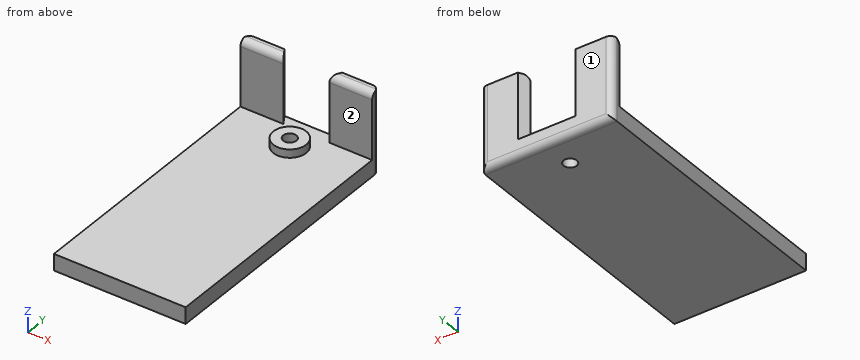
Autodesk Inventor part; units mm, degrees
ref_plane "YZ Plane" through (0, 0, 0) normal (1, 0, 0) x (0, 1, 0)
ref_plane "XZ Plane" through (0, 0, 0) normal (0, 1, 0) x (-1, 0, 0)
ref_plane "XY Plane" through (0, 0, 0) normal (0, 0, 1) x (1, 0, 0)
sketch "Skizze1" plane through (0, 0, 0) normal (0, 0, 1) x (1, 0, 0)
  line L0 (-20, 15) -> (20, 15)
  line L1 (20, 15) -> (20, -67)
  line L2 (20, -67) -> (-20, -67)
  line L3 (-20, -67) -> (-20, 15)
  line L4 (0, -83.4) -> (0, 31.4)
  point P0 (0, 0)
  point P1 (0, 15)
  dimension "d2" = 82
  dimension "d4" = 15
  dimension "d42" = 40
extrude "Extrusion1" add sketch "Skizze1" along normal blind 5
sketch "Skizze2" plane through (0, 0, 5) normal (0, 0, 1) x (1, 0, 0)
  line L0 (20, 15) -> (-20, 15)
  circle A0 centre (0, 5) radius 5
  line L1 (0, -83.4) -> (0, 31.4)
  point P0 (0, 0)
  dimension "d10" = 10
  dimension "d11" = 10
extrude "Extrusion2" add sketch "Skizze2" along normal blind 2.5
sketch "Skizze3" plane through (0, 5, 7.5) normal (0, 0, 1) x (1, 0, 0)
  circle A0 centre (0, 0) radius 5
  circle A1 centre (0, 0) radius 1
  point P0 (0, -5)
  dimension "d15" = 2
hole "Bohrung1" at (0, 5, 7.5) direction (0, 0, -1) diameter 4 end through all
sketch "Skizze6" plane through (0, 0, 5) normal (0, 0, 1) x (1, 0, 0)
  line L0 (20, -67) -> (20, 15)
  line L1 (20, 15) -> (-20, 15)
  circle A0 centre (0, 5) radius 5
  line L2 (-20, -67) -> (20, -67)
  line L3 (-20, 15) -> (-20, -67)
sketch "Skizze7" plane through (0, 0, 5) normal (0, 0, 1) x (1, 0, 0)
  circle A0 centre (0, 5) radius 5
  line L0 (-20, -67) -> (20, -67)
  line L1 (20, -67) -> (20, 15)
  line L2 (20, 15) -> (-20, 15)
  line L3 (-20, 15) -> (-20, -67)
  point P0 (0, 0)
sketch "Skizze9" plane through (0, 0, 5) normal (0, 0, 1) x (1, 0, 0)
  line L0 (20, -67) -> (20, 15)
  line L1 (20, 15) -> (-20, 15)
  line L2 (-20, 15) -> (-20, -67)
  line L3 (20, 15) -> (20, 12)
  line L4 (20, 12) -> (-20, 12)
  line L5 (-20, 12) -> (-20, 15)
  line L6 (-8.7321, 15) -> (-7, 12)
  line L7 (8.7321, 15) -> (7, 12)
  line L8 (8.7321, 15) -> (12.1962, 15) construction
  line L9 (-20, 15) -> (-8.7321, 15)
  line L10 (8.7321, 15) -> (20, 15)
  point P0 (0, 0)
  point P1 (-8.7321, 15)
  dimension "d52" = 3
  dimension "d54" = 120
  dimension "d56" = 13
  dimension "d57" = 13
  dimension "d60" = 120
extrude "Extrusion6" add sketch "Skizze9" along normal blind 20 contours L4 L7 L1 L0 | L4 L2 L1 L6
fillet "Rundung1" radius 2 5 edges at (20, 15, 12.5) (-20, 15, 12.5) (0, 15, 0) (13.5, 12, 25) (-13.5, 12, 25)
properties part number "Gehäuse" material "1.2067 100 Cr 6 (WS)"
Build history of the part. All positions in model axes, mm. Face numbers are marked on the shaded views. A direction names the side the tool comes from. Round coordinates to 2 decimals unless told otherwise and drop trailing zeros. Write each loop counter-clockwise with the first axis right and the second up, starting at its lowest first coordinate (ties: lowest second). Pieces come first, ordered by that corner, then holes. Notation, with made-up numbers: (-15, 48.5) -> (0, 48.5) arc R26 ccw to (0, 75.5) -> close; hole circle Ø10 at (56, 27.25). An arc over 180 degrees is marked (long way). Put each result on its own line as item: value.
Item 1: Tool access for the marked faces 1 and 2: list every direction of +Z, -Z, +X, -X, +Y, -Y with a clear straight run to the whole face (end or side of a thin tool).
Here are the results:
face 1: +Z, -Z, +X, -X, +Y
face 2: +Z, +X, -X, -Y
Item 2: Slice it at B-B, the plane x = 0. Give the cut face in (y, z).
Here are the results:
outline: (-67, 0) -> (3, 0) -> (3, 7.5) -> (0, 7.5) -> (0, 5) -> (-67, 5) -> close; (7, 0) -> (13, 0) arc R2 ccw to (15, 2) -> (15, 5) -> (10, 5) -> (10, 7.5) -> (7, 7.5) -> close
Item 3: Flat gauge pins, fed straight in: P1, Ø10, axis at y = -1, z = 7, coming from the +X side; P2, Ø20, axis at x = 5, y = -36, coming from the +Z side; P3, Ø6.5, axis at x = -16, z = 14, coming from the -Y side; P4, Ø3, axis at x = 0, y = 5, coming from the +Z side. Where does each tip first touch, or does it go through?
Here are the results:
P1: stops at x = 20
P2: stops at z = 5
P3: stops at y = 12
P4: passes through
Item 4: Slice it at A-A, the plane z = 8.75. Give the cut face in (x, y).
Here are the results:
outline: (-20, 12) -> (-7, 12) -> (-8.73, 15) -> (-18, 15) arc R2 ccw to (-20, 13) -> close; (7, 12) -> (20, 12) -> (20, 13) arc R2 ccw to (18, 15) -> (8.73, 15) -> close
Item 5: Slice it at D-D, the plane x = 13. Give the cut face in (y, z), plus the area to 3 significant figures.
Here are the results:
outline: (-67, 0) -> (13, 0) arc R2 ccw to (15, 2) -> (15, 25) -> (14, 25) arc R2 ccw to (12, 23) -> (12, 5) -> (-67, 5) -> close
area: 468 mm^2
Item 6: Slice it at C-C, the plane y = 5. Give the cut face in (x, z), plus the area to 3 significant figures.
Here are the results:
outline: (-20, 0) -> (-2, 0) -> (-2, 7.5) -> (-5, 7.5) -> (-5, 5) -> (-20, 5) -> close; (2, 0) -> (20, 0) -> (20, 5) -> (5, 5) -> (5, 7.5) -> (2, 7.5) -> close
area: 195 mm^2
Item 7: Wall check: probe 1 along Y at (x, z) = (0, 4.25); probe 2 along X at (y, z) = (5, 2.25); probe 3 along Z at (x, y) = (12, -41). Give the ranges that are in metal, low to high. Write a range as from..to.
Here are the results:
probe 1: y = -67..3, 7..15
probe 2: x = -20..-2, 2..20
probe 3: z = 0..5
